```python
from build123d import *

# Parameters (mm, degrees)
SKETCH1_R               = 1.25
BOSS_EXTRUDE1_DEPTH     = 50
F_1_4_28_TAPPED_HOLE1_D = 5.4102


with BuildPart() as part:
    # Sketch1 → Boss-Extrude1 (new body)
    with BuildSketch(Plane.XY):
        Polygon((-7.332348419, -12.7), (7.332348419, -12.7), (14.664696837, 0), (7.332348419, 12.7), (-7.332348419, 12.7), (-14.664696837, 0), align=None)
        with Locations((-7.794228634, 4.5)):
            Circle(SKETCH1_R, mode=Mode.SUBTRACT)
        with Locations((7.794228634, 4.5)):
            Circle(SKETCH1_R, mode=Mode.SUBTRACT)
        with Locations((0, -9)):
            Circle(SKETCH1_R, mode=Mode.SUBTRACT)
    extrude(amount=BOSS_EXTRUDE1_DEPTH)

    # 1/4-28 Tapped Hole1 (through all)
    with Locations(Plane(origin=(0, 12.7, 0), x_dir=(1, 0, 0), z_dir=(0, 1, 0))):
        with Locations((0, -25)):
            Hole(F_1_4_28_TAPPED_HOLE1_D / 2)


solid = part.part
```
Read the model definition and answer for the solid it produces. Units are mm, in the model's axes. Coordinates: 2 decimals unless noted, no trailing zeros. Write each loop counter-clockwise with the first axis right and the second up, starting at its lowest first coordinate (ties: lowest second). Pieces come first, ordered by that corner, then holes. Notation, with made-up numbers: (-21.75, -13) -> (-7.75, -13) arc R16 cw to (-7.75, -2) -> close; hole circle Ø5 at (-14.5, 0). An arc over 180 degrees is marked (long way). Answer as a JSON object with one key per item and string values.
Q1. The part is cut by section A-A on x = 0. Give the vertices of the cut face in (y, z).
The answers:
{"outline": "(-12.7, 0) -> (-10.25, 0) -> (-10.25, 22.29) -> (-12.7, 22.29) -> close; (-12.7, 27.71) -> (-10.25, 27.71) -> (-10.25, 50) -> (-12.7, 50) -> close; (-7.75, 0) -> (12.7, 0) -> (12.7, 22.29) -> (-7.75, 22.29) -> close; (-7.75, 27.71) -> (12.7, 27.71) -> (12.7, 50) -> (-7.75, 50) -> close"}
Q2. The part is cut by section B-B on z = 25. Give the vertices of the cut face in (x, y).
The answers:
{"outline": "(-14.66, 0) -> (-7.33, -12.7) -> (-2.71, -12.7) -> (-2.71, 12.7) -> (-7.33, 12.7) -> close; (2.71, -12.7) -> (7.33, -12.7) -> (14.66, 0) -> (7.33, 12.7) -> (2.71, 12.7) -> close; hole circle Ø2.5 at (-7.79, 4.5); hole circle Ø2.5 at (7.79, 4.5)"}
Q3. Flat-ended cylindrical pins translate along their axes: pin 1 Ø8 at (y, z) = (-10, 38) entering from -X; pin 2 Ø1 at (x, z) = (11.5, 29.5) entering from -Y; pin 3 Ø8 at (y, z) = (6, 8.5) entering from -X. Find the tip coordinate at first contact, or state that the pin passes through.
The answers:
{"pin 1": "stops at x = -11.2", "pin 2": "stops at y = -6.35", "pin 3": "stops at x = -13.51"}
Q4. Consider line 1 (X direction, y = 5.5, z = 25); line 2 (Z direction, x = 0, y = 5.75); line 3 (X direction, y = 5, z = 24.5). Determine where each line is inside the solid, lowest interval first. Write a range as [from, to].
The answers:
{"line 1": "x = [-11.49, -8.54], [-7.04, -2.71], [2.71, 7.04], [8.54, 11.49]", "line 2": "z = [0, 22.29], [27.71, 50]", "line 3": "x = [-11.78, -8.94], [-6.65, -2.66], [2.66, 6.65], [8.94, 11.78]"}
Q5. The part is cut by section C-C on y = 4.5. Give the vertices of the cut face in (x, z), then the cut area to 3 significant figures.
The answers:
{"outline": "(-12.07, 0) -> (-9.04, 0) -> (-9.04, 50) -> (-12.07, 50) -> close; (-6.54, 0) -> (6.54, 0) -> (6.54, 50) -> (-6.54, 50) -> close; (9.04, 0) -> (12.07, 0) -> (12.07, 50) -> (9.04, 50) -> close; hole circle Ø5.41 at (0, 25)", "area": "934 mm2"}
Q6. The part is cut by section D-D on z = 40. Give the vertices of the cut face in (x, y), then the cut area to 3 significant figures.
The answers:
{"outline": "(-14.66, 0) -> (-7.33, -12.7) -> (7.33, -12.7) -> (14.66, 0) -> (7.33, 12.7) -> (-7.33, 12.7) -> close; hole circle Ø2.5 at (-7.79, 4.5); hole circle Ø2.5 at (0, -9); hole circle Ø2.5 at (7.79, 4.5)", "area": "544 mm2"}
Q7. Determine the mould class of faces 1 (the cylindrical face through (-8.07, 3.28, 24.65)), 2 (the flat face through (3, 12.7, 25)), 3 (the flat face through (0, 0, 50)) for opening direction Y: pulls with the +Y half, pulls with the -Y half, needs draft (parallel to the pull), parting line crosses it, or undercut.
The answers:
{"face 1": "undercut", "face 2": "pulls with the +Y half", "face 3": "needs draft"}
